Geometry: final body of the model. Coordinates: model frame, mm. Round coordinates to 2 decimals unless told otherwise and drop trailing zeros. Order: outer loops, then holes, each group sorted by start corner. A loop starts at its lowest first (then second) coordinate and runs counter-clockwise, first axis right, second up. Notation, with made-up numbers: M -17,56 L 13,56 A23 ccw 13,76 Z; hole C 78,77 d11. An arc over 180 degrees is marked long. Return JSON: item names as keys, results as strings. Group by question number.
Q1. Contact query for flat-ended pins moving along their axis: pin 1 (3.5 mm diameter, centred on x = -75, z = -87, fed in from +Y); pin 2 (2.5 mm diameter, centred on x = 1, y = 1.5, fed in from -Z); pin 3 (1.5 mm diameter, centred on x = -1, y = 4, fed in from +Z). Output: stop coordinate, or through.
Q2. Cut plane A-A on x = -51. Output: boundary loops of the cut face in (y, z).
Q3. Cut plane B-B on y = 4.2. Count the separate pieces of the cut face and the enclosed holes in it, and give its area (3 significant figures).
Q4. Ray query, probe 1 along Z at (x, y) = (-75, 3.15); probe 2 along Z at (x, y) = (-64, 3.2). Return the intervals inside material, ascending.
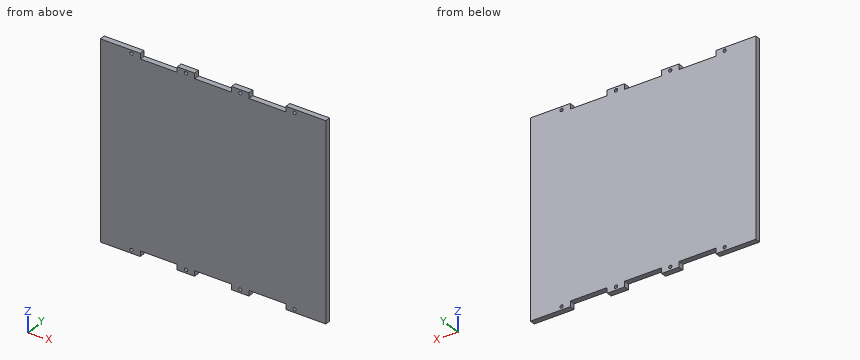
```python
from build123d import *

# Parameters (mm, degrees)
CROQUIS1_W                  = 200
CROQUIS1_H                  = 180
SALIENTE_EXTRUIR1_DEPTH     = 5
CROQUIS4_W                  = 17
CROQUIS4_H                  = 5
CROQUIS4_W_2                = 34
CORTAR_EXTRUIR4_DEPTH       = 135.629120178
SIMETR_A3_COPY_1_SKETCH_W   = 17
SIMETR_A3_COPY_1_SKETCH_H   = 5
SIMETR_A3_COPY_1_SKETCH_W_2 = 34
SIMETR_A3_COPY_1_DEPTH      = 135.629120178
CROQUIS5_R                  = 1.5
CORTAR_EXTRUIR5_DEPTH       = 135.629120178
CROQUIS6_W                  = 17
CROQUIS6_H                  = 5
SALIENTE_EXTRUIR3_DEPTH     = 5
SIMETR_A6_COPY_1_SKETCH_W   = 17
SIMETR_A6_COPY_1_SKETCH_H   = 5
SIMETR_A6_COPY_1_DEPTH      = 5
CROQUIS9_W                  = 3.69
CROQUIS9_H                  = 180
SALIENTE_EXTRUIR7_DEPTH     = 5


with BuildPart() as part:
    # Croquis1 → Saliente-Extruir1 (new body)
    with BuildSketch(Plane(origin=(0, 0, 0), x_dir=(1, 0, 0), z_dir=(0, 1, 0))):
        Rectangle(CROQUIS1_W, CROQUIS1_H)
    extrude(amount=SALIENTE_EXTRUIR1_DEPTH)

    # Croquis4 → Cortar-Extruir4 (cut, through all)
    with BuildSketch(Plane(origin=(0, 5, 0), x_dir=(1, 0, 0), z_dir=(0, 1, 0))):
        with Locations((-91.5, -87.5)):
            Rectangle(CROQUIS4_W, CROQUIS4_H)
        with Locations((-50, -87.5)):
            Rectangle(CROQUIS4_W_2, CROQUIS4_H)
        with Locations((-8.5, -87.5)):
            Rectangle(CROQUIS4_W, CROQUIS4_H)
    cortar_extruir4 = extrude(amount=-CORTAR_EXTRUIR4_DEPTH, mode=Mode.SUBTRACT)

    # Simetría2: Cortar-Extruir4 across plane
    add(cortar_extruir4.mirror(Plane(origin=(0, 0, 0), x_dir=(0, 0, 1), z_dir=(1, 0, 0))), mode=Mode.SUBTRACT)

    # Simetría3: Cortar-Extruir4 across plane
    add(cortar_extruir4.mirror(Plane.XY), mode=Mode.SUBTRACT)

    # Simetría3 copy 1 sketch → Simetría3 copy 1 (cut, through all)
    with BuildSketch(Plane(origin=(0, 5, 0), x_dir=(-1, 0, 0), z_dir=(0, 1, 0))):
        with Locations((-91.5, -87.5)):
            Rectangle(SIMETR_A3_COPY_1_SKETCH_W, SIMETR_A3_COPY_1_SKETCH_H)
        with Locations((-50, -87.5)):
            Rectangle(SIMETR_A3_COPY_1_SKETCH_W_2, SIMETR_A3_COPY_1_SKETCH_H)
        with Locations((-8.5, -87.5)):
            Rectangle(SIMETR_A3_COPY_1_SKETCH_W, SIMETR_A3_COPY_1_SKETCH_H)
    extrude(amount=-SIMETR_A3_COPY_1_DEPTH, mode=Mode.SUBTRACT)

    # Croquis5 → Cortar-Extruir5 (cut, through all)
    with BuildSketch(Plane(origin=(0, 5, 0), x_dir=(1, 0, 0), z_dir=(0, 1, 0))):
        with Locations(Location((-75, -87, 0), (0, 0, 270))):
            Circle(CROQUIS5_R)
        with Locations(Location((-25, -87, 0), (0, 0, 270))):
            Circle(CROQUIS5_R)
        with Locations(Location((25, -87, 0), (0, 0, 270))):
            Circle(CROQUIS5_R)
        with Locations(Location((75, -87, 0), (0, 0, 270))):
            Circle(CROQUIS5_R)
    cortar_extruir5 = extrude(amount=-CORTAR_EXTRUIR5_DEPTH, mode=Mode.SUBTRACT)

    # Simetría4: Cortar-Extruir5 across plane
    add(cortar_extruir5.mirror(Plane.XY), mode=Mode.SUBTRACT)

    # Croquis6 → Saliente-Extruir3 (add, through all)
    with BuildSketch(Plane(origin=(0, 5, 0), x_dir=(1, 0, 0), z_dir=(0, 1, 0))):
        with Locations((91.5, 87.5)):
            Rectangle(CROQUIS6_W, CROQUIS6_H)
    saliente_extruir3 = extrude(amount=-SALIENTE_EXTRUIR3_DEPTH)

    # Simetría5: Saliente-Extruir3 across plane
    add(saliente_extruir3.mirror(Plane(origin=(0, 0, 0), x_dir=(0, 0, 1), z_dir=(1, 0, 0))))

    # Simetría6: Saliente-Extruir3 across plane
    add(saliente_extruir3.mirror(Plane.XY))

    # Simetría6 copy 1 sketch → Simetría6 copy 1 (add, through all)
    with BuildSketch(Plane(origin=(0, 5, 0), x_dir=(-1, 0, 0), z_dir=(0, 1, 0))):
        with Locations((91.5, 87.5)):
            Rectangle(SIMETR_A6_COPY_1_SKETCH_W, SIMETR_A6_COPY_1_SKETCH_H)
    extrude(amount=-SIMETR_A6_COPY_1_DEPTH)

    # Croquis9 → Saliente-Extruir7 (add)
    with BuildSketch(Plane(origin=(0, 5, 0), x_dir=(1, 0, 0), z_dir=(0, 1, 0))):
        with Locations((101.845, 0)):
            Rectangle(CROQUIS9_W, CROQUIS9_H)
    saliente_extruir7 = extrude(amount=-SALIENTE_EXTRUIR7_DEPTH)

    # Simetría7: Saliente-Extruir7 across plane
    add(saliente_extruir7.mirror(Plane(origin=(0, 0, 0), x_dir=(0, 0, 1), z_dir=(1, 0, 0))))


solid = part.part
```
Result sheet:
{
 "1": {"pin 1": "stops at y = 5", "pin 2": "stops at z = -85", "pin 3": "stops at z = 85"},
 "2": {"outline": "M 0,-85 L 5,-85 L 5,85 L 0,85 Z"},
 "3": {"separate pieces": "1", "enclosed holes": "8", "area": "36,300 mm²"},
 "4": {"probe 1": "z = -90 to -88.5, -85.5 to 85.5, 88.5 to 90", "probe 2": "z = -85 to 85"}
}
